Source: CAD feature listing. Evaluate the final solid. Frame: model axes, mm. A direction names the side the tool comes from. Coordinates: 2 decimals unless noted, no trailing zeros. Write each loop counter-clockwise with the first axis right and the second up, starting at its lowest first coordinate (ties: lowest second). Pieces come first, ordered by that corner, then holes. Notation, with made-up numbers: (-37, 21) - (-10, 21) arc R27 ccw to (-10, 60) - close; hole circle Ø8 at (75.5, -9.75). An arc over 180 degrees is marked (long way). One line per question, with ' | ' between items. Start each with the question number.
Q1. Cut plane C-C, the plane y = 13. Return loops of the section in (x, z), plus the area to 3 significant figures.
Q2. Cut plane D-D, the plane z = 52. Return loops of the section in (x, y), plus the area to 3 significant figures.
Q3. Cut plane A-A, the plane z = 125. Return loops of the section in (x, y), plus the area to 3 significant figures.
Q4. Contact query for flat-ended pins moving along their axis: P1, Ø5.5, axis at x = 0, z = 25, coming from the +Y side; P2, Ø4, axis at x = -14.5, z = 46.5, coming from the +Y side; P3, Ø11.5, axis at x = 0, z = 25, coming from the +Y side; P4, Ø8, axis at x = -0.5, z = 123.5, coming from the +Y side. Output: stop coordinate, or through.
Q5. Access query for faces 1 (the face through (0, 3, 20)), 2 (the face through (0, 8, 153)). Directions: +Z, -Z, +X, -X, +Y, -Y. A direction counts if a zero-diameter tool reaches every point of the face in a straight line with its end or side. Return the directions, or none.
Q6. Line query: line 1 (X direction, y = 1, z = 125); line 2 (Z direction, x = -5.5, y = 5.5); line 3 (X direction, y = 3.4, z = 125). Output: solid intervals per line, ascending.
Q7. Cut plane B-B, the plane x = 0. Return loops of the section in (y, z).
Autodesk Inventor part; units mm, degrees
ref_plane "YZ Plane" through (0, 0, 0) normal (1, 0, 0) x (0, 1, 0)
ref_plane "XZ Plane" through (0, 0, 0) normal (0, 1, 0) x (-1, 0, 0)
ref_plane "XY Plane" through (0, 0, 0) normal (0, 0, 1) x (1, 0, 0)
sketch "Sketch3" plane through (0, 0, 0) normal (0, 0, 1) x (1, 0, 0)
  line L0 (-19, 0) -> (19, 0)
  arc A0 (-16, 15.9689) -> (16, 15.9689) centre (0, 20) ccw
  line L1 (0, -4) -> (0, 24)
  line L2 (-26.6, 0) -> (26.6, 0)
  line L3 (-16, 15.9689) -> (-19, 15.9689)
  line L4 (-19, 15.9689) -> (-19, 0)
  line L5 (16, 15.9689) -> (19, 15.9689)
  line L6 (19, 15.9689) -> (19, 0)
  point P0 (0, 0)
  point P1 (-17.5, 15.9689)
  point P2 (17.5, 15.9689)
  dimension "d6" = 16.5
  dimension "d9" = 20
  dimension "d12" = 38
  dimension "d13" = 3
  dimension "d14" = 3
extrude "Extrusion3" add sketch "Sketch3" along normal blind 150
ref_plane "Work Plane1" through (0, 0, 75) normal (0, 0, 1) x (1, 0, 0)
sketch "Sketch4" plane through (0, 0, 0) normal (0, 0, -1) x (-1, 0, 0)
  line L0 (-19, 0) -> (-19, 15.9689)
  line L1 (19, 15.9689) -> (19, 0)
  line L2 (-19, 15.9689) -> (19, 15.9689)
  line L3 (19, 15.9689) -> (19, 0)
  line L4 (19, 0) -> (-19, 0)
  line L5 (-19, 0) -> (-19, 15.9689)
  point P0 (0, 0)
  point P1 (19, 15.9689)
extrude "Extrusion4" add sketch "Sketch4" along normal blind 3
mirror "Mirror1" about plane through (0, 0, 75) normal (0, 0, 1) of "Extrusion4"
fillet "Fillet1" radius 1 12 edges at (-16, 15.9689, 75) (-19, 15.9689, 75) (19, 15.9689, 75) (16, 15.9689, 75) (0, 15.9689, 150) (0, 15.9689, 153) (0, 15.9689, -3) (0, 15.9689, 0) (19, 7.9844, -3) (19, 7.9844, 153) (-19, 7.9844, 153) (-19, 7.9844, -3)
ref_plane "Work Plane2" through (-18, 4.5, -3) normal (0, -1, 0) x (1, 0, 0)
sketch "Sketch5" plane through (-18, 4.5, -3) normal (0, -1, 0) x (1, 0, 0)
  line L0 (-1, 1) -> (-1, 155)
  line L1 (0, 156) -> (36, 156)
  line L2 (36, 0) -> (0, 0)
  point P0 (18, 3)
  point P1 (18, 128)
  point P2 (18, 28)
  dimension "d20" = 19
  dimension "d21" = 100
  dimension "d22" = 28
  dimension "d23" = 28
hole "Hole1" at (0, 4.5, 125) at (0, 4.5, 25) direction (0, -1, 0) diameter 6 end through all counterbore diameter 10 counterbore depth 2.5
properties part number "Disk_Holder_3DPrint"
Reply:
1) outline: (-19, -2) arc R1 ccw to (-18, -3) - (18, -3) arc R1 ccw to (19, -2) - (19, 152) arc R1 ccw to (18, 153) - (-18, 153) arc R1 ccw to (-19, 152) - close; hole (-14.94, 0) - (14.94, 0) - (14.94, 150) - (-14.94, 150) - close | area: 1,440 mm^2
2) outline: (-19, 0) - (19, 0) - (19, 14.97) arc R1 ccw to (18, 15.97) - (16.76, 15.97) arc R1 ccw to (15.8, 15.26) arc R16.5 cw to (-15.8, 15.26) arc R1 ccw to (-16.76, 15.97) - (-18, 15.97) arc R1 ccw to (-19, 14.97) - close | area: 310 mm^2
3) outline: (-19, 0) - (-3, 0) - (-3, 2) - (-5, 2) - (-5, 4.28) arc R16.5 cw to (-15.8, 15.26) arc R1 ccw to (-16.76, 15.97) - (-18, 15.97) arc R1 ccw to (-19, 14.97) - close; (3, 0) - (19, 0) - (19, 14.97) arc R1 ccw to (18, 15.97) - (16.76, 15.97) arc R1 ccw to (15.8, 15.26) arc R16.5 cw to (5, 4.28) - (5, 2) - (3, 2) - close | area: 281 mm^2
4) P1: passes through | P2: stops at y = 15.93 | P3: stops at y = 4.53 | P4: stops at y = 4.1
5) face 1: +Y | face 2: +Z, +X, -X, +Y, -Y
6) line 1: x = -19 to -3, 3 to 19 | line 2: z = -3 to 0, 150 to 153 | line 3: x = -19 to -5, 5 to 19
7) outline: (0, -3) - (14.97, -3) arc R1 ccw to (15.97, -2) - (15.97, -1) arc R1 ccw to (14.97, 0) - (3.5, 0) - (3.5, 20) - (2, 20) - (2, 22) - (0, 22) - close; (0, 28) - (2, 28) - (2, 30) - (3.5, 30) - (3.5, 120) - (2, 120) - (2, 122) - (0, 122) - close; (0, 128) - (2, 128) - (2, 130) - (3.5, 130) - (3.5, 150) - (14.97, 150) arc R1 ccw to (15.97, 151) - (15.97, 152) arc R1 ccw to (14.97, 153) - (0, 153) - close
